from build123d import *

# Parameters (mm, degrees)
SKIZZE1_W                                           = 100
SKIZZE1_H                                           = 50
AUFSATZ_LINEAR_AUSTRAGEN1_DEPTH                     = 200
STIRNSENKUNG_F_R_M8_SENKSCHRAUBE_KOPF_B_D           = 9
STIRNSENKUNG_F_R_M8_SENKSCHRAUBE_KOPF_B_CBORE_D     = 15
STIRNSENKUNG_F_R_M8_SENKSCHRAUBE_KOPF_B_CBORE_DEPTH = 6.5
SPIEGELN3_COPY_1_D                                  = 9
SPIEGELN3_COPY_1_CBORE_D                            = 15
SPIEGELN3_COPY_1_CBORE_DEPTH                        = 6.5
KERNLOCH_F_R_M8_HELICOIL0_D                         = 8.3
KERNLOCH_F_R_M8_HELICOIL0_DEPTH                     = 20
KERNLOCH_F_R_M8_HELICOIL0_TIP                       = 2.493571569
KERNLOCH_F_R_M8_HELICOIL0_2_D                       = 8.3
KERNLOCH_F_R_M8_HELICOIL0_2_DEPTH                   = 20
KERNLOCH_F_R_M8_HELICOIL0_2_TIP                     = 2.493571569
KERNLOCH_F_R_M8_HELICOIL3_D                         = 8.3
KERNLOCH_F_R_M8_HELICOIL3_DEPTH                     = 20
KERNLOCH_F_R_M8_HELICOIL3_TIP                       = 2.493571569
KERNLOCH_F_R_M8_HELICOIL4_D                         = 8.3
KERNLOCH_F_R_M8_HELICOIL4_DEPTH                     = 20
KERNLOCH_F_R_M8_HELICOIL4_TIP                       = 2.493571569


with BuildPart() as part:
    # Skizze1 → Aufsatz-Linear austragen1 (new body)
    with BuildSketch(Plane.XY):
        Rectangle(SKIZZE1_W, SKIZZE1_H)
    extrude(amount=AUFSATZ_LINEAR_AUSTRAGEN1_DEPTH)

    # Stirnsenkung für M8 Senkschraube (Kopf Button)4 (through all)
    with Locations(Plane(origin=(0, 25, 0), x_dir=(1, 0, 0), z_dir=(0, 1, 0))):
        with Locations((-35, -185)):
            stirnsenkung_f_r_m8_senkschraube_kopf_b = CounterBoreHole(STIRNSENKUNG_F_R_M8_SENKSCHRAUBE_KOPF_B_D / 2, STIRNSENKUNG_F_R_M8_SENKSCHRAUBE_KOPF_B_CBORE_D / 2, STIRNSENKUNG_F_R_M8_SENKSCHRAUBE_KOPF_B_CBORE_DEPTH)

    # Spiegeln2: Stirnsenkung für M8 Senkschraube (Kopf Button)4 across plane
    add(stirnsenkung_f_r_m8_senkschraube_kopf_b.mirror(Plane(origin=(0, 0, 0), x_dir=(0, 0, 1), z_dir=(1, 0, 0))), mode=Mode.SUBTRACT)

    # Spiegeln3: Stirnsenkung für M8 Senkschraube (Kopf Button)4 across plane
    add(stirnsenkung_f_r_m8_senkschraube_kopf_b.mirror(Plane.XY.offset(100)), mode=Mode.SUBTRACT)

    # Spiegeln3 copy 1 (through all)
    with Locations(Plane(origin=(0, 25, 200), x_dir=(-1, 0, 0), z_dir=(0, 1, 0))):
        with Locations((-35, -185)):
            CounterBoreHole(SPIEGELN3_COPY_1_D / 2, SPIEGELN3_COPY_1_CBORE_D / 2, SPIEGELN3_COPY_1_CBORE_DEPTH)

    # Kernloch f_r M8 Helicoil0
    with Locations(Plane.ZY.offset(50)):
        with Locations((35, -7.5)):
            Hole(KERNLOCH_F_R_M8_HELICOIL0_D / 2, depth=KERNLOCH_F_R_M8_HELICOIL0_DEPTH)
            with Locations((0, 0, -(KERNLOCH_F_R_M8_HELICOIL0_DEPTH + KERNLOCH_F_R_M8_HELICOIL0_TIP / 2))):  # 118° drill point
                Cone(0, KERNLOCH_F_R_M8_HELICOIL0_D / 2, KERNLOCH_F_R_M8_HELICOIL0_TIP, mode=Mode.SUBTRACT)

    # Kernloch f_r M8 Helicoil0 2
    with Locations(Plane.ZY.offset(50)):
        with Locations((165, -7.5)):
            Hole(KERNLOCH_F_R_M8_HELICOIL0_2_D / 2, depth=KERNLOCH_F_R_M8_HELICOIL0_2_DEPTH)
            with Locations((0, 0, -(KERNLOCH_F_R_M8_HELICOIL0_2_DEPTH + KERNLOCH_F_R_M8_HELICOIL0_2_TIP / 2))):  # 118° drill point
                Cone(0, KERNLOCH_F_R_M8_HELICOIL0_2_D / 2, KERNLOCH_F_R_M8_HELICOIL0_2_TIP, mode=Mode.SUBTRACT)

    # Kernloch für M8 Helicoil3
    with Locations(Plane.XY.offset(200)):
        with Locations((0, 0)):
            Hole(KERNLOCH_F_R_M8_HELICOIL3_D / 2, depth=KERNLOCH_F_R_M8_HELICOIL3_DEPTH)
            with Locations((0, 0, -(KERNLOCH_F_R_M8_HELICOIL3_DEPTH + KERNLOCH_F_R_M8_HELICOIL3_TIP / 2))):  # 118° drill point
                Cone(0, KERNLOCH_F_R_M8_HELICOIL3_D / 2, KERNLOCH_F_R_M8_HELICOIL3_TIP, mode=Mode.SUBTRACT)

    # Kernloch für M8 Helicoil4
    with Locations(Plane(origin=(0, 25, 0), x_dir=(1, 0, 0), z_dir=(0, 1, 0))):
        with Locations((-17.5, -65), (17.5, -65), (17.5, -155), (-17.5, -155)):
            Hole(KERNLOCH_F_R_M8_HELICOIL4_D / 2, depth=KERNLOCH_F_R_M8_HELICOIL4_DEPTH)
            with Locations((0, 0, -(KERNLOCH_F_R_M8_HELICOIL4_DEPTH + KERNLOCH_F_R_M8_HELICOIL4_TIP / 2))):  # 118° drill point
                Cone(0, KERNLOCH_F_R_M8_HELICOIL4_D / 2, KERNLOCH_F_R_M8_HELICOIL4_TIP, mode=Mode.SUBTRACT)


solid = part.part
Can you work these out from the model? Positions are in its coordinate system, mm. A direction names the side the tool comes from. Give positions to 0.01 mm unless a question says otherwise; leave off trailing zeros. Order: outer loops, then holes, each group sorted by start corner. A loop starts at its lowest first (then second) coordinate and runs counter-clockwise, first axis right, second up. Notation, with made-up numbers: M 84.5,1 L 115.5,1 A16 ccw 115.5,21 Z; hole C 0.25,-5 d9. An arc over 180 degrees is marked long. Use one line per item in the form item = value. Start each with the question number.
Item 1: We'd pull the mould along Z, two halves only. Please class faces 4 (the flat face through (-1, 0, 0)), 5 (the flat face through (-1, -25, 99)), 6 (the flat face through (35, 18.5, 10)): +Z half, -Z half, draft (parallel to the pull), parting line (faces both ways), or undercut.
Item 2: If we section it at B-B (x = 35): Write out the boundary of the cut face in (y, z).
Item 3: If we section it at A-A (x = -35): Write out the boundary of the cut face in (y, z), then the cut area to 3 significant figures.
Item 4: For faces 1 (the cylindrical face through (-39.86, -6.253, 31.042)), 2 (the flat face through (-1, 25, 99)), 3 (the cylindrical face through (-40.5, 21.8, 20.1)), which set-ups out of +Z, -Z, +X, -X, +Y, -Y let a thin tool reach every point of the face, with its end or its side?
Item 5: Will these pins go through, and if not, where does the flat tip stop? pin 1 Ø11.5 at (x, z) = (-35, 15) entering from +Y; pin 2 Ø8 at (x, z) = (35, 185) entering from -Y; pin 3 Ø5 at (x, z) = (17.5, 65) entering from +Y.
Item 6: If we section it at C-C (y = 10): State how many separate pieces and enclosed holes the cut face has, then the cut area to 3 significant figures.
Item 7: If I drill on line 1 along X through (y, z) = (10, 65); line 2 along Z through (x, y) = (-17.5, 12.5); line 3 along Z through (x, y) = (35, 2.5), over which ranges is the centre line in solid material (lowest first)?
Outcome:
q1.face_4 = -Z half
q1.face_5 = draft
q1.face_6 = undercut
q2.outline = M -25,0 L 25,0 L 25,7.5 L 18.5,7.5 L 18.5,10.5 L -25,10.5 Z; M -25,19.5 L 18.5,19.5 L 18.5,22.5 L 25,22.5 L 25,177.5 L 18.5,177.5 L 18.5,180.5 L -25,180.5 Z; M -25,189.5 L 18.5,189.5 L 18.5,192.5 L 25,192.5 L 25,200 L -25,200 Z
q3.outline = M -25,0 L 25,0 L 25,7.5 L 18.5,7.5 L 18.5,10.5 L -25,10.5 Z; M -25,19.5 L 18.5,19.5 L 18.5,22.5 L 25,22.5 L 25,177.5 L 18.5,177.5 L 18.5,180.5 L -25,180.5 Z; M -25,189.5 L 18.5,189.5 L 18.5,192.5 L 25,192.5 L 25,200 L -25,200 Z; hole C -7.5,35 d8.3; hole C -7.5,165 d8.3
q3.area = 8,910 mm2
q4.face_1 = -X
q4.face_2 = +Z, -Z, +X, -X, +Y
q4.face_3 = +Y
q5.pin_1 = 18.5
q5.pin_2 = through
q5.pin_3 = 4.01
q6.separate_pieces = 1
q6.enclosed_holes = 8
q6.area = 19,500 mm2
q7.line_1 = -50 to -21.65, -13.35 to 13.35, 21.65 to 50
q7.line_2 = 0 to 60.85, 69.15 to 150.85, 159.15 to 200
q7.line_3 = 0 to 10.5, 19.5 to 180.5, 189.5 to 200
